Could you check a few things on this model? Use its own coordinates, in mm. A direction names the side the tool comes from. Round coordinates to 2 decimals unless told otherwise and drop trailing zeros. Write each loop counter-clockwise with the first axis right and the second up, starting at its lowest first coordinate (ties: lowest second). Pieces come first, ordered by that corner, then holes. Notation, with made-up numbers: (45.25, 28.5) - (82.25, 28.5) arc R23 cw to (82.25, 64.5) - close; hole circle Ø9 at (62.25, -11). An arc over 180 degrees is marked (long way). Write each question's results on one line, items separated by ' | '. Start each with the question number.
(1) On a 3-axis mill with a long thin cutter (end or side, diameter ignored), from which of +Z, -Z, +X, -X, +Y, -Y can I reach the whole of each face in a straight line? I mean faces 5 (the cylindrical face through (4.51, -0.35, 3.44)), 6 (the flat face through (-4, -2, 34)). Say none if no direction works.
(2) Imagine slicing it at C-C on x = 0. Write out the boundary of the cut face in (y, z).
(3) Imagine slicing it at D-D on z = 5. Write out the boundary of the cut face in (x, y), then the cut area to 3 significant figures.
(4) Thinking about a two-plate mould opening in X: for faces 1 (the cylindrical face through (4.51, 0.74, 32.08)), 2 (the flat face through (5, 2, 34)), 3 (the cylindrical face through (-0.86, -4.49, 54.85)), 4 (the flat face through (-5, 2, 34)), which applies, +X half, -X half, draft (parallel to the pull), parting line (faces both ways), or undercut?
(5) Imagine slicing it at B-B on y = 2.75. Write out the boundary of the cut face in (x, z).
(6) Imagine slicing it at A-A on z = 53.5. Write out the boundary of the cut face in (x, y), then the cut area to 3 significant figures.
(7) Please list where these lines run through material, in increasing order: line 1 (Z direction, x = 4.8, y = 0); line 2 (Z direction, x = 0, y = 4.4); line 3 (Y direction, x = 1, z = 16.5). Write a range as [from, to].
```python
from build123d import *

# Parameters (mm, degrees)
SKETCH_1_W          = 10
SKETCH_1_H          = 10
SKETCH_1_W_2        = 8
SKETCH_1_H_2        = 8
EXTRUDE_1_DEPTH     = 68.5
SKETCH_2_R          = 1.6
CUT_EXTRUDE_1_DEPTH = 70.406411808
SKETCH_3_R          = 1.6
CUT_EXTRUDE_2_DEPTH = 70.406411808
SKETCH_4_R          = 1.6
CUT_EXTRUDE_3_DEPTH = 70.406411808


with BuildPart() as part:
    # ｽｹｯﾁ1 → 押し出し-薄板1 (new body)
    with BuildSketch(Plane.XY):
        Rectangle(SKETCH_1_W, SKETCH_1_H)
        Rectangle(SKETCH_1_W_2, SKETCH_1_H_2, mode=Mode.SUBTRACT)
    extrude(amount=EXTRUDE_1_DEPTH)

    # ｽｹｯﾁ2 → ｶｯﾄ - 押し出し1 (cut, through all)
    with BuildSketch(Plane(origin=(0, 5, 0), x_dir=(1, 0, 0), z_dir=(0, 1, 0))):
        with Locations(Location((0, -63.5, 0), (0, 0, 180))):
            Circle(SKETCH_2_R)
        with Locations(Location((0, -53.5, 0), (0, 0, 180))):
            Circle(SKETCH_2_R)
    extrude(amount=-CUT_EXTRUDE_1_DEPTH, mode=Mode.SUBTRACT)

    # ｽｹｯﾁ3 → ｶｯﾄ - 押し出し2 (cut, through all)
    with BuildSketch(Plane(origin=(5, 0, 0), x_dir=(0, 0, -1), z_dir=(1, 0, 0))):
        with Locations(Location((-5, 0, 0), (0, 0, 90))):
            Circle(SKETCH_3_R)
        with Locations(Location((-15, 0, 0), (0, 0, 90))):
            Circle(SKETCH_3_R)
    extrude(amount=-CUT_EXTRUDE_2_DEPTH, mode=Mode.SUBTRACT)

    # ｽｹｯﾁ4 → ｶｯﾄ - 押し出し3 (cut, through all)
    with BuildSketch(Plane(origin=(5, 0, 0), x_dir=(0, 0, -1), z_dir=(1, 0, 0))):
        with Locations(Location((-53.5, 0, 0), (0, 0, 90))):
            Circle(SKETCH_4_R)
        with Locations(Location((-33.5, 0, 0), (0, 0, 90))):
            Circle(SKETCH_4_R)
    extrude(amount=-CUT_EXTRUDE_3_DEPTH, mode=Mode.SUBTRACT)


solid = part.part
```
Response:
1) face 5: +X, -X | face 6: +Z, -Z
2) outline: (-5, 0) - (-4, 0) - (-4, 51.9) - (-5, 51.9) - close; (-5, 55.1) - (-4, 55.1) - (-4, 61.9) - (-5, 61.9) - close; (-5, 65.1) - (-4, 65.1) - (-4, 68.5) - (-5, 68.5) - close; (4, 0) - (5, 0) - (5, 51.9) - (4, 51.9) - close; (4, 55.1) - (5, 55.1) - (5, 61.9) - (4, 61.9) - close; (4, 65.1) - (5, 65.1) - (5, 68.5) - (4, 68.5) - close
3) outline: (-5, -5) - (5, -5) - (5, -1.6) - (4, -1.6) - (4, -4) - (-4, -4) - (-4, -1.6) - (-5, -1.6) - close; (-5, 1.6) - (-4, 1.6) - (-4, 4) - (4, 4) - (4, 1.6) - (5, 1.6) - (5, 5) - (-5, 5) - close | area: 29.6 mm²
4) face 1: draft | face 2: +X half | face 3: undercut | face 4: -X half
5) outline: (-5, 0) - (-4, 0) - (-4, 68.5) - (-5, 68.5) - close; (4, 0) - (5, 0) - (5, 68.5) - (4, 68.5) - close
6) outline: (-5, -5) - (-1.6, -5) - (-1.6, -4) - (-4, -4) - (-4, -1.6) - (-5, -1.6) - close; (-5, 1.6) - (-4, 1.6) - (-4, 4) - (-1.6, 4) - (-1.6, 5) - (-5, 5) - close; (1.6, -5) - (5, -5) - (5, -1.6) - (4, -1.6) - (4, -4) - (1.6, -4) - close; (1.6, 4) - (4, 4) - (4, 1.6) - (5, 1.6) - (5, 5) - (1.6, 5) - close | area: 23.2 mm²
7) line 1: [0, 3.4], [6.6, 13.4], [16.6, 31.9], [35.1, 51.9], [55.1, 68.5] | line 2: [0, 51.9], [55.1, 61.9], [65.1, 68.5] | line 3: [-5, -4], [4, 5]
